```python
from build123d import *

# Parameters (mm, degrees)
SKETCH1_R           = 1.5
SKETCH1_R_2         = 1.75
BOSS_EXTRUDE3_DEPTH = 2
CUT_EXTRUDE1_DEPTH  = 2
FILLET1_R           = 1


with BuildPart() as part:
    # Sketch1 → Boss-Extrude3 (new body)
    with BuildSketch(Plane(origin=(0, 0, 0), x_dir=(1, 0, 0), z_dir=(0, 1, 0))):
        with BuildLine():
            Line((6.048353149, 16.421553647), (2.27592576, 17.351373488))
            ThreePointArc((2.27592576, 17.351373488), (1.69730064, 18.342788524), (1.499767326, 19.473580897))
            ThreePointArc((1.499767326, 19.473580897), (1.49994183, 19.486789936), (1.5, 19.5))
            ThreePointArc((1.5, 19.5), (0, 21), (-1.5, 19.5))
            ThreePointArc((-1.5, 19.5), (-1.49994183, 19.486789936), (-1.499767326, 19.473580897))
            ThreePointArc((-1.499767326, 19.473580897), (-1.69730064, 18.342788524), (-2.27592576, 17.351373488))
            Line((-2.27592576, 17.351373488), (-6.048353149, 16.421553647))
            ThreePointArc((-6.048353149, 16.421553647), (-7.021433788, 17.030507563), (-7.72184627, 17.939976175))
            ThreePointArc((-7.72184627, 17.939976175), (-7.7278303, 17.951753295), (-7.733917816, 17.963477258))
            ThreePointArc((-7.733917816, 17.963477258), (-9.759186613, 18.594576539), (-10.390285893, 16.569307742))
            ThreePointArc((-10.390285893, 16.569307742), (-10.384020417, 16.557678026), (-10.377802301, 16.546022918))
            ThreePointArc((-10.377802301, 16.546022918), (-10.027203946, 15.452957688), (-10.078817505, 14.30620277))
            Line((-10.078817505, 14.30620277), (-12.987027242, 11.729753767))
            ThreePointArc((-12.987027242, 11.729753767), (-14.131642352, 11.81674256), (-15.174477944, 12.296539112))
            ThreePointArc((-15.174477944, 12.296539112), (-15.18524964, 12.304186316), (-15.196088265, 12.31173836))
            ThreePointArc((-15.196088265, 12.31173836), (-17.282661184, 11.929359681), (-16.900282505, 9.842786762))
            ThreePointArc((-16.900282505, 9.842786762), (-16.889330102, 9.835400872), (-16.878407836, 9.827970489))
            ThreePointArc((-16.878407836, 9.827970489), (-16.059995669, 9.023040475), (-15.572773623, 7.983653406))
            Line((-15.572773623, 7.983653406), (-16.950529904, 4.350808657))
            ThreePointArc((-16.950529904, 4.350808657), (-18.004461959, 3.895904243), (-19.150819593, 3.836113127))
            ThreePointArc((-19.150819593, 3.836113127), (-19.163911289, 3.837878533), (-19.177018025, 3.839528576))
            ThreePointArc((-19.177018025, 3.839528576), (-20.846886356, 2.531270285), (-19.538628065, 0.861401954))
            ThreePointArc((-19.538628065, 0.861401954), (-19.5254978, 0.859951908), (-19.512373542, 0.858448461))
            ThreePointArc((-19.512373542, 0.858448461), (-18.413635928, 0.526053428), (-17.499194975, -0.167854741))
            Line((-17.499194975, -0.167854741), (-17.030870442, -4.024854283))
            ThreePointArc((-17.030870442, -4.024854283), (-17.752676308, -4.917438785), (-18.739939265, -5.503120145))
            ThreePointArc((-18.739939265, -5.503120145), (-18.752351812, -5.50764097), (-18.764724063, -5.512270933))
            ThreePointArc((-18.764724063, -5.512270933), (-19.635341096, -7.446702628), (-17.700909402, -8.317319661))
            ThreePointArc((-17.700909402, -8.317319661), (-17.688609259, -8.312501675), (-17.676289619, -8.307733764))
            ThreePointArc((-17.676289619, -8.307733764), (-16.548934104, -8.09144612), (-15.416761648, -8.280909389))
            Line((-15.416761648, -8.280909389), (-13.209643805, -11.478471612))
            ThreePointArc((-13.209643805, -11.478471612), (-13.433966457, -12.604255849), (-14.035964693, -13.581654911))
            ThreePointArc((-14.035964693, -13.581654911), (-14.044854525, -13.591426301), (-14.053657958, -13.601275602))
            ThreePointArc((-14.053657958, -13.601275602), (-13.925575823, -15.718725712), (-11.808125713, -15.590643577))
            ThreePointArc((-11.808125713, -15.590643577), (-11.799473508, -15.5806613), (-11.790780767, -15.570714303))
            ThreePointArc((-11.790780767, -15.570714303), (-10.893070914, -14.855292874), (-9.802534018, -14.496907492))
            Line((-9.802534018, -14.496907492), (-6.362246966, -16.302509425))
            ThreePointArc((-6.362246966, -16.302509425), (-6.037696789, -17.403589796), (-6.116519761, -18.548796214))
            ThreePointArc((-6.116519761, -18.548796214), (-6.119850325, -18.561579661), (-6.12306818, -18.574391943))
            ThreePointArc((-6.12306818, -18.574391943), (-5.02562895, -20.389778166), (-3.210242727, -19.292338936))
            ThreePointArc((-3.210242727, -19.292338936), (-3.207220575, -19.279479189), (-3.204146136, -19.266631842))
            ThreePointArc((-3.204146136, -19.266631842), (-2.741736452, -18.215971056), (-1.942663979, -17.391838795))
            Line((-1.942663979, -17.391838795), (1.942663979, -17.391838795))
            ThreePointArc((1.942663979, -17.391838795), (2.741736452, -18.215971056), (3.204146136, -19.266631842))
            ThreePointArc((3.204146136, -19.266631842), (3.207137832, -19.279498812), (3.210242727, -19.292338936))
            ThreePointArc((3.210242727, -19.292338936), (5.02562895, -20.389778166), (6.12306818, -18.574391943))
            ThreePointArc((6.12306818, -18.574391943), (6.11976794, -18.561600739), (6.116519761, -18.548796214))
            ThreePointArc((6.116519761, -18.548796214), (6.037696789, -17.403589796), (6.362246966, -16.302509425))
            Line((6.362246966, -16.302509425), (9.802534018, -14.496907492))
            ThreePointArc((9.802534018, -14.496907492), (10.893070914, -14.855292874), (11.790780767, -15.570714303))
            ThreePointArc((11.790780767, -15.570714303), (11.799409362, -15.580717128), (11.808125713, -15.590643577))
            ThreePointArc((11.808125713, -15.590643577), (13.925575823, -15.718725712), (14.053657958, -13.601275602))
            ThreePointArc((14.053657958, -13.601275602), (14.044791371, -13.591483251), (14.035964693, -13.581654911))
            ThreePointArc((14.035964693, -13.581654911), (13.433966458, -12.604255849), (13.209643805, -11.478471612))
            Line((13.209643805, -11.478471612), (15.416761648, -8.280909389))
            ThreePointArc((15.416761648, -8.280909389), (16.548934104, -8.09144612), (17.676289619, -8.307733764))
            ThreePointArc((17.676289619, -8.307733764), (17.688578405, -8.312580919), (17.700909402, -8.317319661))
            ThreePointArc((17.700909402, -8.317319661), (19.635341096, -7.446702628), (18.764724063, -5.512270933))
            ThreePointArc((18.764724063, -5.512270933), (18.752322358, -5.507720745), (18.739939265, -5.503120145))
            ThreePointArc((18.739939265, -5.503120145), (17.752676308, -4.917438785), (17.030870442, -4.024854283))
            Line((17.030870442, -4.024854283), (17.499194975, -0.167854741))
            ThreePointArc((17.499194975, -0.167854741), (18.413635928, 0.526053428), (19.512373542, 0.858448461))
            ThreePointArc((19.512373542, 0.858448461), (19.525507306, 0.859867402), (19.538628065, 0.861401954))
            ThreePointArc((19.538628065, 0.861401954), (20.846886356, 2.531270285), (19.177018025, 3.839528576))
            ThreePointArc((19.177018025, 3.839528576), (19.163922282, 3.837794208), (19.150819593, 3.836113127))
            ThreePointArc((19.150819593, 3.836113127), (18.004461959, 3.895904243), (16.950529904, 4.350808657))
            Line((16.950529904, 4.350808657), (15.572773623, 7.983653406))
            ThreePointArc((15.572773623, 7.983653406), (16.059995669, 9.023040475), (16.878407836, 9.827970489))
            ThreePointArc((16.878407836, 9.827970489), (16.889377792, 9.835330464), (16.900282505, 9.842786762))
            ThreePointArc((16.900282505, 9.842786762), (17.282661184, 11.929359681), (15.196088265, 12.31173836))
            ThreePointArc((15.196088265, 12.31173836), (15.185298562, 12.304116759), (15.174477944, 12.296539112))
            ThreePointArc((15.174477944, 12.296539112), (14.131642352, 11.81674256), (12.987027242, 11.729753767))
            Line((12.987027242, 11.729753767), (10.078817505, 14.30620277))
            ThreePointArc((10.078817505, 14.30620277), (10.027203946, 15.452957688), (10.377802301, 16.546022918))
            ThreePointArc((10.377802301, 16.546022918), (10.384095364, 16.557637845), (10.390285893, 16.569307742))
            ThreePointArc((10.390285893, 16.569307742), (9.759186613, 18.594576539), (7.733917816, 17.963477258))
            ThreePointArc((7.733917816, 17.963477258), (7.727905944, 17.95171444), (7.72184627, 17.939976175))
            ThreePointArc((7.72184627, 17.939976175), (7.021433788, 17.030507563), (6.048353149, 16.421553647))
        make_face()
        with Locations(Location((0, -9, 0), (0, 0, 270))):
            Circle(SKETCH1_R, mode=Mode.SUBTRACT)
        with Locations(Location((-7.794228634, -4.5, 0), (0, 0, 270))):
            Circle(SKETCH1_R, mode=Mode.SUBTRACT)
        with Locations(Location((0, 0, 0), (0, 0, 270))):
            Circle(SKETCH1_R_2, mode=Mode.SUBTRACT)
        with Locations(Location((7.794228634, -4.5, 0), (0, 0, 270))):
            Circle(SKETCH1_R, mode=Mode.SUBTRACT)
        with Locations(Location((-7.794228634, 4.5, 0), (0, 0, 270))):
            Circle(SKETCH1_R, mode=Mode.SUBTRACT)
        with Locations(Location((0, 9, 0), (0, 0, 270))):
            Circle(SKETCH1_R, mode=Mode.SUBTRACT)
        with Locations(Location((7.794228634, 4.5, 0), (0, 0, 270))):
            Circle(SKETCH1_R, mode=Mode.SUBTRACT)
    extrude(amount=BOSS_EXTRUDE3_DEPTH)

    # Sketch3 → Cut-Extrude1 (cut)
    with BuildSketch(Plane(origin=(0, 2, 0), x_dir=(1, 0, 0), z_dir=(0, 1, 0))):
        with BuildLine():
            Line((-3, 14.186260959), (-3, 11.618950039))
            ThreePointArc((-3, 11.618950039), (-10.392304845, 6), (-11.562305899, -3.211398808))
            Line((-11.562305899, -3.211398808), (-13.785662375, -4.495054268))
            ThreePointArc((-13.785662375, -4.495054268), (-12.557368355, 7.25), (-3, 14.186260959))
        make_face()
        with BuildLine():
            Line((3, 14.186260959), (3, 11.618950039))
            ThreePointArc((3, 11.618950039), (10.392304845, 6), (11.562305899, -3.211398808))
            Line((11.562305899, -3.211398808), (13.785662375, -4.495054268))
            ThreePointArc((13.785662375, -4.495054268), (12.557368355, 7.25), (3, 14.186260959))
        make_face()
        with BuildLine():
            Line((10.785662375, -9.691206691), (8.562305899, -8.407551231))
            ThreePointArc((8.562305899, -8.407551231), (0, -12), (-8.562305899, -8.407551231))
            Line((-8.562305899, -8.407551231), (-10.785662375, -9.691206691))
            ThreePointArc((-10.785662375, -9.691206691), (0, -14.5), (10.785662375, -9.691206691))
        make_face()
    extrude(amount=-CUT_EXTRUDE1_DEPTH, mode=Mode.SUBTRACT)

    # Fillet1
    fillet1_edges = [part.edges().sort_by_distance(p)[0] for p in [
        (-8.562305899, 1, 8.407551231),
        (8.562305899, 1, 8.407551231),
        (10.785662375, 1, 9.691206691),
        (-10.785662375, 1, 9.691206691),
        (11.562305899, 1, 3.211398808),
        (3, 1, -11.618950039),
        (3, 1, -14.186260959),
        (13.785662375, 1, 4.495054268),
        (-3, 1, -11.618950039),
        (-11.562305899, 1, 3.211398808),
        (-13.785662375, 1, 4.495054268),
        (-3, 1, -14.186260959),
    ]]
    fillet(fillet1_edges, radius=FILLET1_R)


solid = part.part
```
Geometry: final body of the model. Coordinates: model frame, mm. A direction names the side the tool comes from. Coordinates: 2 decimals unless noted, no trailing zeros. Order: outer loops, then holes, each group sorted by start corner. A loop starts at its lowest first (then second) coordinate and runs counter-clockwise, first axis right, second up. Notation, with made-up numbers: (23, -8.75) - (53, -8.75) arc R10 ccw to (53, 0.25) - close; hole circle Ø8 at (-36.5, -10). An arc over 180 degrees is marked (long way). Return JSON: item names as keys, results as strings. Group by question number.
1. Pull-direction query (X, two-part tool) for faces 4 (the face through (17.262, 0.986, 2.123)), 5 (the face through (-3.2, 0.99, -11.77)), 6 (the face through (4, 2, -1)); classes: pulls with the +X half, pulls with the -X half, needs draft (parallel to the pull), parting line crosses it, or undercut.
2. Cut plane B-B (y = 0.9). Count the separate pieces of the cut face and the enclosed holes in it, plus the area to 3 significant figures.
3. Pin query (flat end, axial travel): pin 1 (0.6 mm diameter, centred on y = 0.5, z = -12.5, fed in from -X); pin 2 (1 mm diameter, centred on x = -11, y = 1.5, fed in from +Z). Return the tip coordinate at first contact, or that it passes through.
4. Material intervals for line 1 along X through (y, z) = (0.6, -4.5); line 2 along X through (y, z) = (1.6, 10); line 3 along X through (y, z) = (1.1, -9.5), sorted ascending. Write a range as [from, to].
5. Cut plane A-A (z = -9). Output: boundary loops of the cut face in (x, y).
6. Set-up query: faces 1 (the face through (-8.598, 0.986, 8.655)), 2 (the face through (-2.75, 0.99, 18.23)), 3 (the face through (-4.1, 1, -16.9)). Return all of +Z, -Z, +X, -X, +Y, -Y with unobstructed straight access to the full face (end or side cutting, diameter ignored); none if empty.
Resolved:
{
 "1": {"face 4": "pulls with the +X half", "face 5": "undercut", "face 6": "needs draft"},
 "2": {"separate pieces": "1", "enclosed holes": "10", "area": "884 mm²"},
 "3": {"pin 1": "stops at x = -17.04", "pin 2": "stops at z = 15.28"},
 "4": {"line 1": "x = [-16.89, -13.78], [-11.12, -9.29], [-6.29, 6.29], [9.29, 11.12], [13.78, 16.89]", "line 2": "x = [-14.23, -10.16], [-6.63, -1.12], [1.12, 6.63], [10.16, 14.23]", "line 3": "x = [-16.47, -10.95], [-7.33, -1.41], [1.41, 7.33], [10.95, 16.47]"},
 "5": {"outline": "(-16.04, 0) - (-11.37, 0) - (-11.37, 2) - (-16.04, 2) - close; (-7.94, 0) - (-1.5, 0) - (-1.5, 2) - (-7.94, 2) - close; (1.5, 0) - (7.94, 0) - (7.94, 2) - (1.5, 2) - close; (11.37, 0) - (16.04, 0) - (16.04, 2) - (11.37, 2) - close"},
 "6": {"face 1": "+Y, -Y", "face 2": "+Z, +Y, -Y", "face 3": "-Z, +Y, -Y"}
}
